Check sheet for the modelled part. Datum: model origin and axes. Units: mm. Face numbers are marked on the shaded views. A direction names the side the tool comes from. Coordinates: 2 decimals unless noted, no trailing zeros. Loops run counter-clockwise (first coordinate to the right, second up) from the corner with the lowest first, then second, coordinate; pieces in that order, holes last. Notation, with made-up numbers: (30.5, -6) -> (68.5, -6) arc R17 ccw to (68.5, 1) -> close; hole circle Ø10 at (-28.5, -5.75). An arc over 180 degrees is marked (long way). Use CSV: the item, a comma, the result in double quotes.
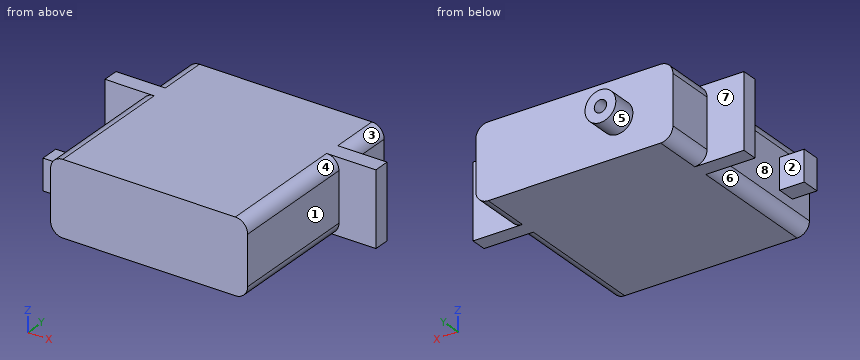
```python
from build123d import *

# Parameters (mm, degrees)
SKETCH1_W                = 40.64
SKETCH1_H                = 40.64
BOSS_EXTRUDE1_DEPTH      = 15.24
SKETCH2_R                = 3.175
BOSS_EXTRUDE2_DEPTH      = 5.08
SKETCH3_R                = 1.27
CUT_EXTRUDE1_DEPTH       = 5.08
FILLET2_R                = 2.54
SKETCH4_W                = 6.35
SKETCH4_H                = 3.81
BOSS_EXTRUDE3_DEPTH      = 5.08
SKETCH5_W                = 15.24
SKETCH5_H                = 3.302
BOSS_EXTRUDE4_DEPTH      = 7.62
BOSS_EXTRUDE4_DEPTH_BACK = 2.54
SKETCH6_W                = 15.24
SKETCH6_H                = 3.302
BOSS_EXTRUDE5_DEPTH      = 7.62
BOSS_EXTRUDE5_DEPTH_BACK = 2.54


with BuildPart() as part:
    # Sketch1 → Boss-Extrude1 (new body)
    with BuildSketch(Plane.XY):
        with Locations((21.271438127, 20.32)):
            Rectangle(SKETCH1_W, SKETCH1_H)
    extrude(amount=BOSS_EXTRUDE1_DEPTH)

    # Sketch2 → Boss-Extrude2 (add)
    with BuildSketch(Plane(origin=(0, 40.64, 0), x_dir=(1, 0, 0), z_dir=(0, 1, 0))):
        with Locations((12.381438127, -7.62)):
            Circle(SKETCH2_R)
    extrude(amount=BOSS_EXTRUDE2_DEPTH)

    # Sketch3 → Cut-Extrude1 (cut)
    with BuildSketch(Plane(origin=(0, 45.72, 0), x_dir=(1, 0, 0), z_dir=(0, 1, 0))):
        with Locations((12.381438127, -7.62)):
            Circle(SKETCH3_R)
    extrude(amount=-CUT_EXTRUDE1_DEPTH, mode=Mode.SUBTRACT)

    # Fillet2
    fillet2_edges = [part.edges().sort_by_distance(p)[0] for p in [
        (41.591438127, 20.32, 15.24),
        (0.951438127, 20.32, 15.24),
        (41.591438127, 20.32, 0),
        (0.951438127, 20.32, 0),
    ]]
    fillet(fillet2_edges, radius=FILLET2_R)

    # Sketch4 → Boss-Extrude3 (add)
    with BuildSketch(Plane.ZY.offset(-0.951438127)):
        with Locations((7.62, 6.985)):
            Rectangle(SKETCH4_W, SKETCH4_H)
    extrude(amount=BOSS_EXTRUDE3_DEPTH)

    # Sketch5 → Boss-Extrude4 (add, two sides)
    with BuildSketch(Plane.ZY.offset(-0.951438127)) as boss_extrude4_sk:
        with Locations((7.62, 28.829)):
            Rectangle(SKETCH5_W, SKETCH5_H)
    extrude(amount=BOSS_EXTRUDE4_DEPTH)
    extrude(boss_extrude4_sk.sketch, amount=-BOSS_EXTRUDE4_DEPTH_BACK)

    # Sketch6 → Boss-Extrude5 (add, two sides)
    with BuildSketch(Plane(origin=(41.591438127, 0, 0), x_dir=(0, 0, -1), z_dir=(1, 0, 0))) as boss_extrude5_sk:
        with Locations((-7.62, 28.829)):
            Rectangle(SKETCH6_W, SKETCH6_H)
    extrude(amount=BOSS_EXTRUDE5_DEPTH)
    extrude(boss_extrude5_sk.sketch, amount=-BOSS_EXTRUDE5_DEPTH_BACK)


solid = part.part
```
1) Cross-section at C-C on x = 35. Record the boundary of the cut face in (y, z).
Answer below:
outline,"(0, 0) -> (40.64, 0) -> (40.64, 15.24) -> (0, 15.24) -> close"
2) Cross-section at B-B on y = 8. Record the boundary of the cut face in (x, z) (3 decimals), and give its area (3 significant figures).
Answer below:
outline,"(-4.129, 4.445) -> (0.951, 4.445) -> (0.951, 2.54) arc R2.54 ccw to (3.491, 0) -> (39.051, 0) arc R2.54 ccw to (41.591, 2.54) -> (41.591, 12.7) arc R2.54 ccw to (39.051, 15.24) -> (3.491, 15.24) arc R2.54 ccw to (0.951, 12.7) -> (0.951, 10.795) -> (-4.129, 10.795) -> close"
area,"646 mm²"
3) Thickness scan on line 1 along X through (y, z) = (44.3, 7.62); line 2 along Y through (x, z) = (0.5, 14.75); line 3 along X through (y, z) = (9, 2.5). Record the ranges inside material, lowest first. Write a range as from..to.
Answer below:
line 1,"x = 9.21..11.11, 13.65..15.56"
line 2,"y = 27.18..30.48"
line 3,"x = 0.95..41.59"
4) Access from +Z, -Z, +X, -X, +Y, -Y to the whole of each face (thin tool, end or side, straight path). Record for the marked faces 1, 2, 3, 4 and 5.
Answer below:
face 1,"+Z, -Z, +X, -Y"
face 2,"+Z, -Z, -X"
face 3,"+Z, +X, +Y"
face 4,"+Z, +X, -Y"
face 5,"+Y"
5) Draft check along Y on the marked faces 6, 7 and 8. Enter one of: released by +Y, released by -Y, zero draft, split by the parting line, or undercut.
Answer below:
face 6,"zero draft"
face 7,"released by +Y"
face 8,"undercut"
6) Cross-section at D-D on y = 37.5. Record the boundary of the cut face in (x, z), and give its area (3 significant figures).
Answer below:
outline,"(0.95, 2.54) arc R2.54 ccw to (3.49, 0) -> (39.05, 0) arc R2.54 ccw to (41.59, 2.54) -> (41.59, 12.7) arc R2.54 ccw to (39.05, 15.24) -> (3.49, 15.24) arc R2.54 ccw to (0.95, 12.7) -> close"
area,"614 mm²"
7) Cross-section at A-A on z = 7.62. Record the boundary of the cut face in (x, y), and give its area (3 significant figures).
Answer below:
outline,"(-6.67, 27.18) -> (0.95, 27.18) -> (0.95, 8.89) -> (-4.13, 8.89) -> (-4.13, 5.08) -> (0.95, 5.08) -> (0.95, 0) -> (41.59, 0) -> (41.59, 27.18) -> (49.21, 27.18) -> (49.21, 30.48) -> (41.59, 30.48) -> (41.59, 40.64) -> (15.56, 40.64) -> (15.56, 45.72) -> (13.65, 45.72) -> (13.65, 40.64) -> (11.11, 40.64) -> (11.11, 45.72) -> (9.21, 45.72) -> (9.21, 40.64) -> (0.95, 40.64) -> (0.95, 30.48) -> (-6.67, 30.48) -> close"
area,"1,740 mm²"
8) Go/stop test with flat-tipped pins: pin 1 Ø5 at (x, z) = (4, 9) entering from -Y; pin 2 Ø3 at (x, z) = (-0.5, 7) entering from +Y; pin 3 Ø8 at (y, z) = (37, 5.5) entering from +X; pin 4 Ø4 at (x, y) = (-2, 6) entering from -Z (3 decimals). Record where each tip stops, or that it passes through.
Answer below:
pin 1,"stops at y = 0"
pin 2,"stops at y = 40.64"
pin 3,"stops at x = 41.59"
pin 4,"stops at z = 4.445"
